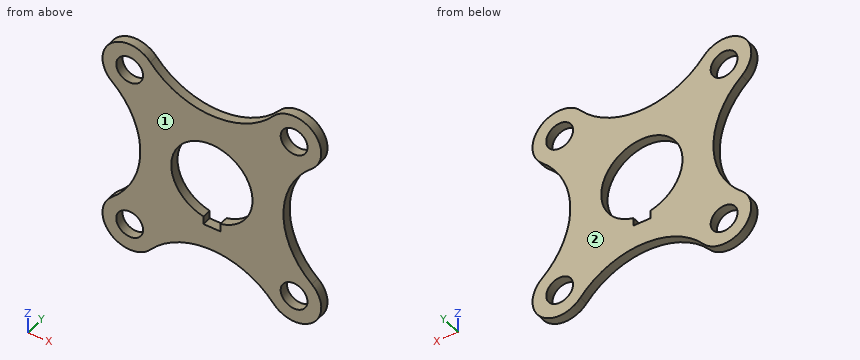
from build123d import *

# Parameters (mm, degrees)
SKETCH1_R           = 2.6
BOSS_EXTRUDE1_DEPTH = 2.54
SKETCH2_R           = 3.75
SKETCH2_R_2         = 2.6
CUT_EXTRUDE1_DEPTH  = 44.322547245


with BuildPart() as part:
    # Sketch1 → Boss-Extrude1 (new body)
    with BuildSketch(Plane(origin=(0, 0, 0), x_dir=(1, 0, 0), z_dir=(0, 1, 0))):
        with BuildLine():
            ThreePointArc((-17.206636662, 27.922333563), (-28.354981926, 28.354981926), (-27.922333563, 17.206636662))
            ThreePointArc((-27.922333563, 17.206636662), (-20, 0), (-27.922333563, -17.206636662))
            ThreePointArc((-27.922333563, -17.206636662), (-28.354981926, -28.354981926), (-17.206636662, -27.922333563))
            ThreePointArc((-17.206636662, -27.922333563), (0, -20), (17.206636662, -27.922333563))
            ThreePointArc((17.206636662, -27.922333563), (28.354981926, -28.354981926), (27.922333563, -17.206636662))
            ThreePointArc((27.922333563, -17.206636662), (20, 0), (27.922333563, 17.206636662))
            ThreePointArc((27.922333563, 17.206636662), (28.354981926, 28.354981926), (17.206636662, 27.922333563))
            ThreePointArc((17.206636662, 27.922333563), (0, 20), (-17.206636662, 27.922333563))
        make_face()
        with Locations(Location((22.980970389, 22.980970389, 0), (0, 0, 270))):
            Circle(SKETCH1_R, mode=Mode.SUBTRACT)
        with Locations(Location((22.980970389, -22.980970389, 0), (0, 0, 270))):
            Circle(SKETCH1_R, mode=Mode.SUBTRACT)
        with Locations(Location((-22.980970389, -22.980970389, 0), (0, 0, 270))):
            Circle(SKETCH1_R, mode=Mode.SUBTRACT)
        with Locations(Location((-22.980970389, 22.980970389, 0), (0, 0, 270))):
            Circle(SKETCH1_R, mode=Mode.SUBTRACT)
        with BuildLine():
            Line((2.353261567, 13.359444444), (-2.353261567, 13.359444444))
            Line((-2.353261567, 13.359444444), (-2.353261567, 11.113016606))
            ThreePointArc((-2.353261567, 11.113016606), (0, -11.359444444), (2.353261567, 11.113016606))
            Line((2.353261567, 11.113016606), (2.353261567, 13.359444444))
        make_face(mode=Mode.SUBTRACT)
    extrude(amount=BOSS_EXTRUDE1_DEPTH)

    # Sketch2 → Cut-Extrude1 (cut, through all)
    # profile 1 of 4: a face of its own
    with BuildSketch(Plane(origin=(0, 2.54, 0), x_dir=(1, 0, 0), z_dir=(0, 1, 0))):
        with Locations(Location((-22.980970389, 22.980970389, 0), (0, 0, 270))):
            Circle(SKETCH2_R)
        with Locations((-22.980970389, 22.980970389)):
            Circle(SKETCH2_R_2, mode=Mode.SUBTRACT)
    # profile 2 of 4: a face of its own
    with BuildSketch(Plane(origin=(0, 2.54, 0), x_dir=(1, 0, 0), z_dir=(0, 1, 0))):
        with Locations(Location((22.980970389, 22.980970389, 0), (0, 0, 270))):
            Circle(SKETCH2_R)
        with Locations((22.980970389, 22.980970389)):
            Circle(SKETCH2_R_2, mode=Mode.SUBTRACT)
    # profile 3 of 4: a face of its own
    with BuildSketch(Plane(origin=(0, 2.54, 0), x_dir=(1, 0, 0), z_dir=(0, 1, 0))):
        with Locations(Location((22.980970389, -22.980970389, 0), (0, 0, 270))):
            Circle(SKETCH2_R)
        with Locations((22.980970389, -22.980970389)):
            Circle(SKETCH2_R_2, mode=Mode.SUBTRACT)
    # profile 4 of 4: a face of its own
    with BuildSketch(Plane(origin=(0, 2.54, 0), x_dir=(1, 0, 0), z_dir=(0, 1, 0))):
        with Locations(Location((-22.980970389, -22.980970389, 0), (0, 0, 270))):
            Circle(SKETCH2_R)
        with Locations((-22.980970389, -22.980970389)):
            Circle(SKETCH2_R_2, mode=Mode.SUBTRACT)
    extrude(amount=-CUT_EXTRUDE1_DEPTH, mode=Mode.SUBTRACT)


solid = part.part
Model file for the job. Use its own axes, mm. Face numbers are marked on the shaded views. Give positions to 0.01 mm unless a question says otherwise; leave off trailing zeros. Order: outer loops, then holes, each group sorted by start corner. A loop starts at its lowest first (then second) coordinate and runs counter-clockwise, first axis right, second up. Notation, with made-up numbers: (27.25, 1) -> (85.25, 1) arc R21 ccw to (85.25, 31) -> close; hole circle Ø8 at (12.5, 76.25). An arc over 180 degrees is marked (long way). Use CSV: the item, a comma, the result in double quotes.
1. Drop flat-ended pins along their axis: pin 1 (0.7 mm diameter, centred on y = 1, z = -12, fed in from +X); pin 2 (7 mm diameter, centred on x = 22.98, z = -22.98, fed in from +Y); pin 3 (8 mm diameter, centred on x = -11.5, z = 24.5, fed in from -Y); pin 4 (1.5 mm diameter, centred on x = -7, y = 1.5, fed in from -Z). Give the stop position or say it passes through.
Outcome:
pin 1,"x = 23.66"
pin 2,"through"
pin 3,"y = 0"
pin 4,"z = -21.37"
2. Mould opens along Y. For the marked faces 1 and 2 say: +Y half, -Y half, draft (parallel to the pull), parting line (faces both ways), or undercut.
Outcome:
face 1,"-Y half"
face 2,"+Y half"
3. Band-saw the part on D-D, the plane z = 13. Give the cut face in (x, y), then the cut area to 3 significant figures.
Outcome:
outline,"(-24.1, 0) -> (24.1, 0) -> (24.1, 2.54) -> (-24.1, 2.54) -> close"
area,"122 mm²"
4. Band-saw the part on B-B, the plane z = 0. Give the cut face in (x, y), then the cut area to 3 significant figures.
Outcome:
outline,"(-20, 0) -> (-11.36, 0) -> (-11.36, 2.54) -> (-20, 2.54) -> close; (11.36, 0) -> (20, 0) -> (20, 2.54) -> (11.36, 2.54) -> close"
area,"43.9 mm²"
5. Band-saw the part on A-A, the plane x = 0. Give the cut face in (y, z).
Outcome:
outline,"(0, -20) -> (2.54, -20) -> (2.54, -13.36) -> (0, -13.36) -> close; (0, 11.36) -> (2.54, 11.36) -> (2.54, 20) -> (0, 20) -> close"
6. Drill centre lines: line 1 along Z through (x, y) = (26, 0.65); line 2 along Z through (x, y) = (22.5, 1.5); line 3 along Z through (x, y) = (9, 0.9). Where is each one in solid material? Low to high. Write a range as from..to.
Outcome:
line 1,"-29.96..-25.21, -20.76..-15.35, 15.35..20.76, 25.21..29.96"
line 2,"-30.57..-26.7, -19.26..-10.34, 10.34..19.26, 26.7..30.57"
line 3,"-21.87..-6.93, 6.93..21.87"
7. Band-saw the part on C-C, the plane y = 0.8. Give the cut face in (x, z).
Outcome:
outline,"(-27.92, -17.21) arc R7.6 ccw (long way) to (-17.21, -27.92) arc R22.65 cw to (17.21, -27.92) arc R7.6 ccw (long way) to (27.92, -17.21) arc R22.65 cw to (27.92, 17.21) arc R7.6 ccw (long way) to (17.21, 27.92) arc R22.65 cw to (-17.21, 27.92) arc R7.6 ccw (long way) to (-27.92, 17.21) arc R22.65 cw to start; hole circle Ø7.5 at (-22.98, -22.98); hole circle Ø7.5 at (-22.98, 22.98); hole (-2.35, -13.36) -> (2.35, -13.36) -> (2.35, -11.11) arc R11.36 ccw (long way) to (-2.35, -11.11) -> close; hole circle Ø7.5 at (22.98, -22.98); hole circle Ø7.5 at (22.98, 22.98)"
